Design review of the part built by this model. Coordinates are the model's own, in mm. Round coordinates to 2 decimals unless told otherwise and drop trailing zeros. Loops run counter-clockwise (first coordinate to the right, second up) from the corner with the lowest first, then second, coordinate; pieces in that order, holes last. Notation, with made-up numbers: (29.25, -5) - (81.25, -5) arc R19 cw to (81.25, 10) - close; hole circle Ø9 at (18, -25). An arc over 180 degrees is marked (long way). Return JSON: item names as keys, results as strings. Group by question number.
(1) Clearance check with a flat-ended pin moving along its axis: pin 1 (3 mm diameter, centred on x = 0, z = -15.5, fed in from +Y). State where the tip first meets the part, or that it passes through.
(2) We need section A-A, the plane z = -15.5. Write out the cut boundary in (x, y).
(3) We need section D-D, the plane y = 0.35. Write out the cut boundary in (x, z), and give its area (3 significant figures).
(4) We need section B-B, the plane x = 0. Write out the cut boundary in (y, z), and give its area (3 significant figures).
(5) The part is to be moulded in two halves that separate along X. For faces 1 (the cylindrical face through (0.46, 0.69, 16.61)), 2 (the cylindrical face through (-0.36, 0.69, -14.355)), 3 (the cylindrical face through (-2.43, 1.23, -17.9)), 4 (the cylindrical face through (2.4, 1.23, -17.93)), say which applies: pulls with the +X half, pulls with the -X half, needs draft (parallel to the pull), parting line crosses it, or undercut.
(6) Wall thickness on L1, parallel to Z at x = 0, y = 0.4; L2, parallel to X at y = 0.55, z = -15.5; L3, parallel to Z at x = 0.95, y = 1.6: over which ranges is each line inside the solid? List them lowest first. Write a range as [from, to].
(7) We need section C-C, the plane y = 2. Write out the cut boundary in (x, z).
Autodesk Inventor part; units mm, degrees
ref_plane "YZ Plane" through (0, 0, 0) normal (1, 0, 0) x (0, 1, 0)
ref_plane "XZ Plane" through (0, 0, 0) normal (0, 1, 0) x (-1, 0, 0)
ref_plane "XY Plane" through (0, 0, 0) normal (0, 0, 1) x (1, 0, 0)
sketch "Эскиз1" plane through (0, 0, 0) normal (0, 1, 0) x (-1, 0, 0)
  line L0 (-1, 18.5) -> (1, 18.5)
  line L1 (3, 16.5) -> (3, -16.5)
  line L2 (1, -18.5) -> (-1, -18.5)
  line L3 (-3, -16.5) -> (-3, 16.5)
  line L4 (-3, 18.5) -> (3, -18.5) construction
  line L5 (3, 18.5) -> (-3, -18.5) construction
  arc A0 (3, 16.5) -> (1, 18.5) centre (1, 16.5) ccw
  arc A1 (-1, 18.5) -> (-3, 16.5) centre (-1, 16.5) ccw
  arc A2 (1, -18.5) -> (3, -16.5) centre (1, -16.5) ccw
  arc A3 (-3, -16.5) -> (-1, -18.5) centre (-1, -16.5) ccw
  circle A4 centre (0, 15.5) radius 2.3
  line L6 (0, 0) -> (0, 8.5528) construction
  line L7 (3, 0) -> (-3, 0) construction
  circle A5 centre (0, -15.5) radius 2.3
  dimension "d0" = 6
  dimension "d1" = 2
  dimension "d2" = 2
  dimension "d3" = 4.6
  dimension "d4" = 3
  dimension "d5" = 15.5
extrude "Выдавливание1" add sketch "Эскиз1" along normal blind 2.5 contours L0 A0 L1 A2 L2 A3 L3 A1 | A4 | A5
sketch "Эскиз2" plane through (0, 2.5, 0) normal (0, 1, 0) x (1, 0, 0)
  circle A0 centre (0, -15.5) radius 2.3
  circle A1 centre (0, 15.5) radius 2.3
  point P0 (0, 0)
hole "Отверстие1" at (0, 2.5, 15.5) at (0, 2.5, -15.5) direction (0, -1, 0) diameter 2.4 depth 4 countersink diameter 4.6 countersink angle 90
properties part number "кронштейн wemos"
Solutions:
{
 "1": {"pin 1": "y = 1.7"},
 "2": {"outline": "(-3, 0) - (-1.2, 0) - (-1.2, 1.4) - (-2.3, 2.5) - (-3, 2.5) - close; (1.2, 0) - (3, 0) - (3, 2.5) - (2.3, 2.5) - (1.2, 1.4) - close"},
 "3": {"outline": "(-3, -16.5) arc R2 ccw to (-1, -18.5) - (1, -18.5) arc R2 ccw to (3, -16.5) - (3, 16.5) arc R2 ccw to (1, 18.5) - (-1, 18.5) arc R2 ccw to (-3, 16.5) - close; hole circle Ø2.4 at (0, -15.5); hole circle Ø2.4 at (0, 15.5)", "area": "210 mm^2"},
 "4": {"outline": "(0, -18.5) - (2.5, -18.5) - (2.5, -17.8) - (1.4, -16.7) - (0, -16.7) - close; (0, -14.3) - (1.4, -14.3) - (2.5, -13.2) - (2.5, 13.2) - (1.4, 14.3) - (0, 14.3) - close; (0, 16.7) - (1.4, 16.7) - (2.5, 17.8) - (2.5, 18.5) - (0, 18.5) - close", "area": "78.1 mm^2"},
 "5": {"face 1": "undercut", "face 2": "undercut", "face 3": "pulls with the -X half", "face 4": "pulls with the +X half"},
 "6": {"L1": "[-18.5, -16.7], [-14.3, 14.3], [16.7, 18.5]", "L2": "[-3, -1.2], [1.2, 3]", "L3": "[-18.5, -16.53], [-14.47, 14.47], [16.53, 18.5]"},
 "7": {"outline": "(-3, -16.5) arc R2 ccw to (-1, -18.5) - (1, -18.5) arc R2 ccw to (3, -16.5) - (3, 16.5) arc R2 ccw to (1, 18.5) - (-1, 18.5) arc R2 ccw to (-3, 16.5) - close; hole circle Ø3.6 at (0, -15.5); hole circle Ø3.6 at (0, 15.5)"}
}
